Geometry: final body of the model. Coordinates: model frame, mm. A direction names the side the tool comes from. Give positions to 0.01 mm unless a question says otherwise; leave off trailing zeros. Write each loop counter-clockwise with the first axis right and the second up, starting at its lowest first coordinate (ties: lowest second). Pieces come first, ordered by that corner, then holes.
Q1. Cut plane D-D on x = 29. Return the cut outline in (y, z), plus the area to 3 significant figures.
Q2. Draft query along Z for faces 6 (the face through (12.84, 41.56, -10.28)), 7 (the face through (41.91, 29.24, -4.83)), 8 (the face through (0, 34, -10)). Return one class per face: pulls with the +Z half, pulls with the -Z half, needs draft (parallel to the pull), parting line crosses it, or undercut.
Q3. Cut plane C-C on y = 11. Return the cut outline in (x, z) (3 decimals).
Q4. Cut plane B-B on x = 43.5. Return the cut outline in (y, z).
Q5. Line query: L1, parallel to Y at x = 29.5, z = -2.25; L2, parallel to X at y = 31, z = -2.5 (3 decimals); L3, parallel to Y at x = -0.5, z = -17.5. Output: solid intervals per line, ascending.
Q6. Cut plane A-A on z = -17.75. Return the cut outline in (x, y) (1 decimal), plus the area to 3 significant figures.
Q7. Pin query (flat end, axial travel): pin 1 (3 mm diameter, centred on y = 15.5, z = -2, fed in from -X); pin 2 (2 mm diameter, centred on y = 34, z = -10, fed in from +X) (3 decimals); pin 3 (7 mm diameter, centred on x = 44.5, z = -11, fed in from -Y). Return the tip coordinate at first contact, or that it passes through.
Q8. Reachability of faces 1 (the face through (40.005, 14, -10)), 2 (the face through (46.546, 29, -10)), 3 (the face through (14.037, 38.846, -9.011)), 4 (the face through (-3, 30.531, -10)), 5 (the face through (43, 30.531, -10)) from +Z, -Z, +X, -X, +Y, -Y: full face, straight path, thin tool, end or side. Return the list, or none.
```python
from build123d import *

# Parameters (mm, degrees)
SKETCH1_W           = 40.005
SKETCH1_H           = 19.812
BOSS_EXTRUDE1_DEPTH = 37.7444
SKETCH2_R           = 4.1275
BOSS_EXTRUDE2_DEPTH = 2.2352
SKETCH3_R           = 2.8575
BOSS_EXTRUDE3_DEPTH = 3.2004
BOSS_EXTRUDE4_START = -27.9908
BOSS_EXTRUDE4_DEPTH = 2.54


with BuildPart() as part:
    # Sketch1 → Boss-Extrude1 (new body)
    with BuildSketch(Plane(origin=(0, 0, 0), x_dir=(1, 0, 0), z_dir=(0, 1, 0))):
        with Locations((20.0025, 9.906)):
            Rectangle(SKETCH1_W, SKETCH1_H)
    extrude(amount=BOSS_EXTRUDE1_DEPTH)

    # Sketch2 → Boss-Extrude2 (add)
    with BuildSketch(Plane(origin=(0, 37.7444, 0), x_dir=(1, 0, 0), z_dir=(0, 1, 0))):
        with Locations(Location((10.0076, 9.906, 0), (0, 0, 90))):
            Circle(SKETCH2_R)
    extrude(amount=BOSS_EXTRUDE2_DEPTH)

    # Sketch3 → Boss-Extrude3 (add)
    with BuildSketch(Plane(origin=(0, 39.9796, 0), x_dir=(1, 0, 0), z_dir=(0, 1, 0))):
        with Locations(Location((10.0076, 9.906, 0), (0, 0, 270))):
            Circle(SKETCH3_R)
    extrude(amount=BOSS_EXTRUDE3_DEPTH)

    # Sketch4 → Boss-Extrude4 (add)
    with BuildSketch(Plane.XZ.offset(BOSS_EXTRUDE4_START)):
        with BuildLine():
            Line((0, 0), (-6.5405, 0))
            Line((-6.5405, 0), (-6.5405, -3.3147))
            Line((-6.5405, -3.3147), (-5.652024704, -3.3147))
            ThreePointArc((-5.652024704, -3.3147), (-1.905, -4.9022), (-5.652024704, -6.4897))
            Line((-5.652024704, -6.4897), (-6.5405, -6.4897))
            Line((-6.5405, -6.4897), (-6.5405, -13.3223))
            Line((-6.5405, -13.3223), (-5.652024704, -13.3223))
            ThreePointArc((-5.652024704, -13.3223), (-1.905, -14.9098), (-5.652024704, -16.4973))
            Line((-5.652024704, -16.4973), (-6.5405, -16.4973))
            Line((-6.5405, -16.4973), (-6.5405, -19.812))
            Line((-6.5405, -19.812), (0, -19.812))
            Line((0, -19.812), (0, 0))
        make_face()
        with BuildLine():
            Line((46.5455, -16.4973), (46.5455, -19.812))
            Line((46.5455, -19.812), (40.005, -19.812))
            Line((40.005, -19.812), (40.005, 0))
            Line((40.005, 0), (46.5455, 0))
            Line((46.5455, 0), (46.5455, -3.3147))
            Line((46.5455, -3.3147), (45.657024704, -3.3147))
            ThreePointArc((45.657024704, -3.3147), (41.91, -4.9022), (45.657024704, -6.4897))
            Line((45.657024704, -6.4897), (46.5455, -6.4897))
            Line((46.5455, -6.4897), (46.5455, -13.3223))
            Line((46.5455, -13.3223), (45.657024704, -13.3223))
            ThreePointArc((45.657024704, -13.3223), (41.91, -14.9098), (45.657024704, -16.4973))
            Line((45.657024704, -16.4973), (46.5455, -16.4973))
        make_face()
    extrude(amount=-BOSS_EXTRUDE4_DEPTH)


solid = part.part
```
Data:
1. outline: (0, -19.81) - (37.74, -19.81) - (37.74, 0) - (0, 0) - close
1. area: 748 mm2
2. face 6: parting line crosses it
2. face 7: undercut
2. face 8: needs draft
3. outline: (0, -19.812) - (40.005, -19.812) - (40.005, 0) - (0, 0) - close
4. outline: (27.99, -19.81) - (30.53, -19.81) - (30.53, -17.03) - (27.99, -17.03) - close; (27.99, -12.79) - (30.53, -12.79) - (30.53, -7.02) - (27.99, -7.02) - close; (27.99, -2.78) - (30.53, -2.78) - (30.53, 0) - (27.99, 0) - close
5. L1: y = 0 to 37.74
5. L2: x = 0 to 40.005
5. L3: y = 27.99 to 30.53
6. outline: (-6.5, 28) - (0, 28) - (0, 0) - (40, 0) - (40, 28) - (46.5, 28) - (46.5, 30.5) - (40, 30.5) - (40, 37.7) - (0, 37.7) - (0, 30.5) - (-6.5, 30.5) - close
6. area: 1,540 mm2
7. pin 1: stops at x = 0
7. pin 2: stops at x = 40.005
7. pin 3: stops at y = 27.99
8. face 1: +Z, -Z, +X, -Y
8. face 2: +Z, -Z, +X, +Y, -Y
8. face 3: +Y
8. face 4: +Z, -Z, -X, +Y
8. face 5: +Z, -Z, +X, +Y
